Build history of the part. All positions in model axes, mm. A direction names the side the tool comes from. Give positions to 0.01 mm unless a question says otherwise; leave off trailing zeros. Order: outer loops, then holes, each group sorted by start corner. A loop starts at its lowest first (then second) coordinate and runs counter-clockwise, first axis right, second up. Notation, with made-up numbers: (56.5, 80.25) - (111.5, 80.25) arc R17 cw to (111.5, 89.25) - close; hole circle Ø10 at (-10, -28.75). An arc over 180 degrees is marked (long way). Use a Markdown table: item, result. Add a question column.
(1) Which spindle directions (+Z, -Z, +X, -X, +Y, -Y) get a long thin tool onto all of the face, cutting with end or side? Do faces 1 (the face through (11.667, 33, 1)), 2 (the face through (23.333, 32, 1)), 3 (the face through (0, 3, 1)). Say none if no direction does.
(2) Flat gauge pins, fed straight in: pin 1 (0.9 mm diameter, centred on x = 30, z = 1.5, fed in from +Y); pin 2 (0.9 mm diameter, centred on x = 25.5, z = 1, fed in from -Y); pin 3 (0.9 mm diameter, centred on y = 28, z = 1, fed in from +X). Where does each tip first touch, or does it go through?
(3) Slice it at A-A (y = 34). Write the cut outline in (x, z), then the cut area to 3 significant figures.
(4) Wall check: line 1 (Y direction, x = 31, z = 0.9); line 2 (Y direction, x = 20.5, z = 2.15); line 3 (X direction, y = 11, z = 0.6). Give the ranges that are in metal, low to high.
(5) Slice it at B-B (x = 32). Write the cut outline in (y, z).
from build123d import *

# Parameters (mm, degrees)
F4_DEPTH = 3
F6_DEPTH = 4.5


# Not quite as in the source:
# - a fillet or chamfer that OpenCascade refuses, or shapes differently, is made with other operations: its cross-section is extruded or revolved along the edge and cut away or added


with BuildPart() as f4:
    # F3 (on Top) → F4 (new body)
    with BuildSketch(Plane.XY):
        with BuildLine():
            ThreePointArc((0, 1), (0.2928932188, 0.2928932188), (1, 0))
            Line((1, 0), (34, 0))
            ThreePointArc((34, 0), (34.7071067812, 0.2928932188), (35, 1))
            Line((35, 1), (35, 4))
            ThreePointArc((35, 4), (34.7071067812, 4.7071067812), (34, 5))
            Line((34, 5), (24.3333333333, 5))
            ThreePointArc((24.3333333333, 5), (23.6262265521, 5.2928932188), (23.3333333333, 6))
            Line((23.3333333333, 6), (23.3333333333, 59))
            ThreePointArc((23.3333333333, 59), (23.0404401145, 59.7071067812), (22.3333333333, 60))
            Line((22.3333333333, 60), (12.6666666667, 60))
            ThreePointArc((12.6666666667, 60), (11.9595598855, 59.7071067812), (11.6666666667, 59))
            Line((11.6666666667, 59), (11.6666666667, 6))
            ThreePointArc((11.6666666667, 6), (11.3737734479, 5.2928932188), (10.6666666667, 5))
            Line((10.6666666667, 5), (1, 5))
            ThreePointArc((1, 5), (0.2928932188, 4.7071067812), (0, 4))
            Line((0, 4), (0, 1))
        make_face()
    extrude(amount=F4_DEPTH)

    # F5 (on face) → F6 (join)
    with BuildSketch(Plane.XZ):
        with BuildLine():
            ThreePointArc((17.5, 0), (18.5606601718, 0.4393398282), (19, 1.5))
            ThreePointArc((19, 1.5), (18.5606601718, 2.5606601718), (17.5, 3))
            ThreePointArc((17.5, 3), (16, 1.5), (17.5, 0))
        make_face()
    extrude(amount=F6_DEPTH)

    # F7: fillet of radius 0.5 on 1 edges, made by hand

    # F7_s1 → F7_t2 (revolve, cut)
    with BuildSketch(Plane.YZ.offset(17.5)):
        with BuildLine():
            ThreePointArc((-4, 0), (-4.3535533906, 0.1464466094), (-4.5, 0.5))
            Line((-4.5, 0.5), (-4.5, 0))
            Line((-4.5, 0), (-4, 0))
        make_face()
    revolve(axis=Axis((17.5, -4.5, 1.5), (0, 1, 0)), mode=Mode.SUBTRACT)


solid = f4.part
Solution:
| question | item | result |
|---|---|---|
| 1 | face 1 | +Z, -Z, -X, +Y |
| 1 | face 2 | +Z, -Z, +X, +Y |
| 1 | face 3 | +Z, -Z, -X, +Y, -Y |
| 2 | pin 1 | y = 5 |
| 2 | pin 2 | y = 0 |
| 2 | pin 3 | x = 23.33 |
| 3 | outline | (11.67, 0) - (23.33, 0) - (23.33, 3) - (11.67, 3) - close |
| 3 | area | 35.0 mm2 |
| 4 | line 1 | 0 to 5 |
| 4 | line 2 | 0 to 60 |
| 4 | line 3 | 11.67 to 23.33 |
| 5 | outline | (0, 0) - (5, 0) - (5, 3) - (0, 3) - close |
